Check sheet for the modelled part. Datum: model origin and axes. Units: mm. Face numbers are marked on the shaded views. A direction names the side the tool comes from. Round coordinates to 2 decimals unless told otherwise and drop trailing zeros. Order: outer loops, then holes, each group sorted by start corner. A loop starts at its lowest first (then second) coordinate and runs counter-clockwise, first axis right, second up. Notation, with made-up numbers: (-38.5, 68) -> (-4.5, 68) arc R13 cw to (-4.5, 82) -> close; hole circle Ø2 at (33.25, -10.75). An arc over 180 degrees is marked (long way). Answer in a Markdown table with one row per item.
```python
from build123d import *

# Parameters (mm, degrees)
BOSS_EXTRUDE1_DEPTH = 2.5
SKETCH2_R           = 2.5
CUT_EXTRUDE1_DEPTH  = 3.5


with BuildPart() as part:
    # Sketch1 → Boss-Extrude1 (new body)
    with BuildSketch(Plane(origin=(0, 0, 0), x_dir=(1, 0, 0), z_dir=(0, 1, 0))):
        with BuildLine():
            Line((-6, 25), (-7.5, 0))
            ThreePointArc((-7.5, 0), (0, -7.5), (7.5, 0))
            Line((7.5, 0), (6, 25))
            ThreePointArc((6, 25), (0, 31), (-6, 25))
        make_face()
    extrude(amount=BOSS_EXTRUDE1_DEPTH)

    # Sketch2 → Cut-Extrude1 (cut, through all)
    with BuildSketch(Plane(origin=(0, 2.5, 0), x_dir=(1, 0, 0), z_dir=(0, 1, 0))):
        Circle(SKETCH2_R)
        with BuildLine():
            Line((2.75, 24), (2.75, 10))
            ThreePointArc((2.75, 10), (0, 7.25), (-2.75, 10))
            Line((-2.75, 10), (-2.75, 24))
            ThreePointArc((-2.75, 24), (0, 26.75), (2.75, 24))
        make_face()
    extrude(amount=-CUT_EXTRUDE1_DEPTH, mode=Mode.SUBTRACT)


solid = part.part
```
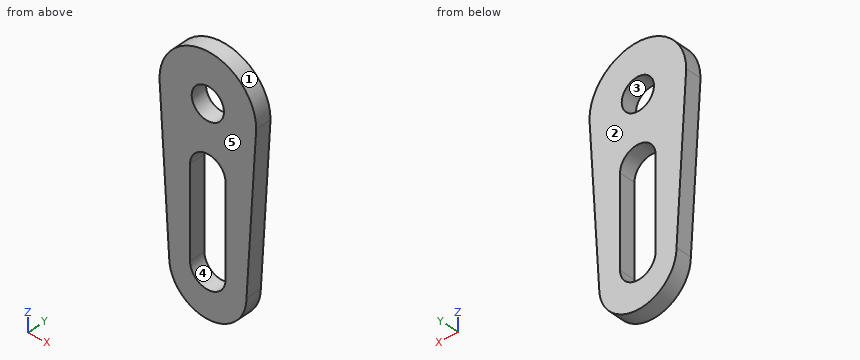
(1) Section check C-C on y = 1.1. Record the boundary of the cut face in (x, z), plus the area to 3 significant figures.
Solutions:
| item | result |
|---|---|
| outline | (-7.5, 0) -> (-6, -25) arc R6 ccw to (6, -25) -> (7.5, 0) arc R7.5 ccw to start; hole (-2.75, -24) arc R2.75 ccw to (2.75, -24) -> (2.75, -10) arc R2.75 ccw to (-2.75, -10) -> close; hole circle Ø5 at (0, 0) |
| area | 362 mm^2 |
(2) Section check D-D on z = -22.5. Record the boundary of the cut face in (x, y), plus the area to 3 significant figures.
Solutions:
| item | result |
|---|---|
| outline | (-6.15, 0) -> (-2.75, 0) -> (-2.75, 2.5) -> (-6.15, 2.5) -> close; (2.75, 0) -> (6.15, 0) -> (6.15, 2.5) -> (2.75, 2.5) -> close |
| area | 17.0 mm^2 |
(3) Scan lines: probe 1 along Z at (x, y) = (0, 1.85); probe 2 along Z at (x, y) = (-1.25, 0.9); probe 3 along X at (y, z) = (2.05, 4.5). Record each from-to range of solid material in increasing order. Write a range as from..to.
Solutions:
| item | result |
|---|---|
| probe 1 | -31..-26.75, -7.25..-2.5, 2.5..7.5 |
| probe 2 | -30.87..-26.45, -7.55..-2.17, 2.17..7.4 |
| probe 3 | -6..6 |
(4) Section check B-B on x = 0. Record the boundary of the cut face in (y, z), plus the area to 3 significant figures.
Solutions:
| item | result |
|---|---|
| outline | (0, -31) -> (2.5, -31) -> (2.5, -26.75) -> (0, -26.75) -> close; (0, -7.25) -> (2.5, -7.25) -> (2.5, -2.5) -> (0, -2.5) -> close; (0, 2.5) -> (2.5, 2.5) -> (2.5, 7.5) -> (0, 7.5) -> close |
| area | 35.0 mm^2 |
(5) Draft check along X on the marked faces 1, 2 and 3. Enter one of: pulls with the +X half, pulls with the -X half, needs draft (parallel to the pull), parting line crosses it, or undercut.
Solutions:
| item | result |
|---|---|
| face 1 | parting line crosses it |
| face 2 | needs draft |
| face 3 | undercut |
(6) Section check A-A on z = -14. Record the boundary of the cut face in (x, y).
Solutions:
| item | result |
|---|---|
| outline | (-6.66, 0) -> (-2.75, 0) -> (-2.75, 2.5) -> (-6.66, 2.5) -> close; (2.75, 0) -> (6.66, 0) -> (6.66, 2.5) -> (2.75, 2.5) -> close |
(7) Tool access check on the marked faces 4 and 5. Record the directions out of +Z, -Z, +X, -X, +Y, -Y that give a thin tool (end or side, any length) a straight path to the whole face; none if there is none.
Solutions:
| item | result |
|---|---|
| face 4 | +Y, -Y |
| face 5 | +Z, -Z, +X, -X, -Y |
(8) Depth check by flat-ended pin: pin 1 Ø1.2 at (y, z) = (1.5, -20.5) entering from -X. Enter the tip coordinate at first touch or a pass-through.
Solutions:
| item | result |
|---|---|
| pin 1 | x = -6.31 |
